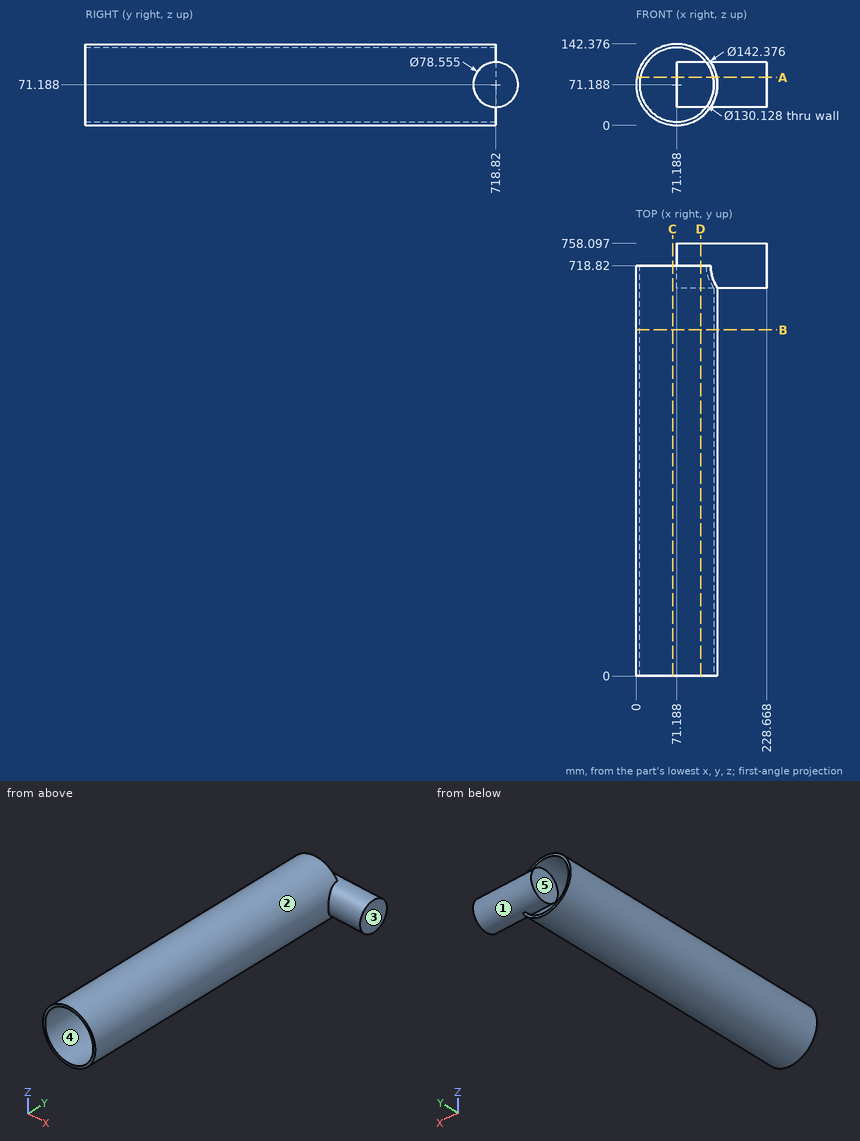
Input: dimensioned drawing with shaded views. Units: mm. Origin: part minimum x, y, z. A direction names the side the tool comes from. Coordinates: 2 decimals unless noted, no trailing zeros. Loops run counter-clockwise (first coordinate to the right, second up) from the corner with the lowest first, then second, coordinate; pieces in that order, holes last. Notation, with made-up numbers: M -5.5,-31 L 17.5,-31 A14 cw 17.5,-23 Z; hole C 10,72.25 d6. An arc over 180 degrees is marked long. Use a Markdown table: item, result. Add a question column.
1) Pin query (flat end, axial travel): P1, Ø10, axis at y = 255, z = 32.5, coming from the +X side; P2, Ø1, axis at y = 375, z = 98, coming from the -X side; P3, Ø10, axis at x = 76, z = 80.5, coming from the +Y side; P4, Ø6, axis at x = 147, y = 609, coming from the +Z side. Return the tip coordinate at first contact, or that it passes through.
2) Draft query along Z for the marked faces 1, 2 and 3. Return one class per face: +Z half, -Z half, draft (parallel to the pull), parting line (faces both ways), or undercut.
3) Set-up query: the marked faces 4 and 5. Return all of +Z, -Z, +X, -X, +Y, -Y with unobstructed straight access to the full face (end or side cutting, diameter ignored); none if empty.
4) Section B-B, the plane y = 606.5. Return the cut outline in (x, z) (1 decimal).
5) Section A-A, the plane z = 84. Return the cut outline in (x, y), plus the area to 3 significant figures.
6) Section D-D, the plane x = 113. Return the cut outline in (y, z) (1 decimal), plus the area to 3 significant figures.
7) Line query: L1, parallel to Z at x = 69.5, y = 199.5 (1 decimal); L2, parallel to Y at x = 194.5, z = 69; L3, parallel to X at y = 533.5, z = 25 (1 decimal). Output: solid intervals per line, ascending. Write a range as from..to.
8) Section C-C, the plane x = 64. Return the cut outline in (y, z).
Answer below:
| question | item | result |
|---|---|---|
| 1 | P1 | x = 133.9 |
| 1 | P2 | x = 5.04 |
| 1 | P3 | y = 757.86 |
| 1 | P4 | through |
| 2 | face 1 | undercut |
| 2 | face 2 | parting line |
| 2 | face 3 | draft |
| 3 | face 4 | -Y |
| 3 | face 5 | +Y, -Y |
| 4 | outline | C 71.2,71.2 d142.4; hole C 71.2,71.2 d130.1 |
| 5 | outline | M 1.16,0 L 7.4,0 L 7.4,718.82 L 1.16,718.82 Z; M 71.19,681.69 L 134.98,681.69 L 134.98,0 L 141.21,0 L 141.21,681.69 L 228.67,681.69 L 228.67,755.95 L 71.19,755.95 Z |
| 5 | area | 20,400 mm2 |
| 6 | outline | M 0,13.6 L 718.8,13.6 L 718.8,21.3 L 0,21.3 Z; M 0,121 L 718.8,121 L 718.8,128.8 L 0,128.8 Z; C 718.8,71.2 d78.6 |
| 6 | area | 16,000 mm2 |
| 7 | L1 | 0..6.1, 136.2..142.4 |
| 7 | L2 | 679.6..758.04 |
| 7 | L3 | 17..25.4, 117..125.4 |
| 8 | outline | M 0,0.36 L 718.82,0.36 L 718.82,6.52 L 0,6.52 Z; M 0,135.85 L 718.82,135.85 L 718.82,142.01 L 0,142.01 Z |
